from build123d import *

# Parameters (mm, degrees)
F0_R     = 3.175
F1_DEPTH = 35.56
F2_R     = 4.7625
F3_DEPTH = 3.81
F4_R     = 1.25


with BuildPart() as f1:
    # F0 (on Top) → F1 (new body)
    with BuildSketch(Plane.XY):
        Circle(F0_R)
    extrude(amount=-F1_DEPTH)

    # F2 (on Top) → F3 (join)
    with BuildSketch(Plane.XY):
        Circle(F2_R)
    extrude(amount=-F3_DEPTH)

    # F4
    f4_edges = [f1.edges().sort_by_distance(p)[0] for p in [
        (-3.175, 0, -35.56),
    ]]
    fillet(f4_edges, radius=F4_R)


solid = f1.part
Design review of the part built by this model. Coordinates are the model's own, in mm. A direction names the side the tool comes from. Round coordinates to 2 decimals unless told otherwise and drop trailing zeros. Order: outer loops, then holes, each group sorted by start corner. A loop starts at its lowest first (then second) coordinate and runs counter-clockwise, first axis right, second up. Notation, with made-up numbers: M 64,-19 L 110,-19 A3 ccw 110,-14 Z; hole C -23,51.5 d1. An arc over 180 degrees is marked long. Answer as CSV lines item,"result". Start each with the question number.
1) Add section C-C (z = -30). Give the boundary of the cut face in (x, y) (3 decimals), then the cut area to 3 significant figures.
2) Wall thickness on line 1 along Z through (x, y) = (0.25, 4); line 2 along X through (y, z) = (-2, -12.5); line 3 along X through (y, z) = (-1, -33): over which ranges is each line inside the solid? List them lowest first. Write a range as [from, to].
3) Tool access review of faces 1 (the face through (0, 0, 0)), 2 (the face through (-0.69, -3.1, -18.85)): name each direction out of +Z, -Z, +X, -X, +Y, -Y from which nothing blocks a thin tool from reaching the whole face with its end or side.
4) Add section D-D (z = -2.5). Give the boundary of the cut face in (x, y) (1 decimal).
5) For pin 1 Ø1.5 at (y, z) = (-1.5, -5.5) entering from -X; pin 2 Ø1.5 at (x, z) = (2, -22) entering from +Y; pin 3 Ø2 at (y, z) = (2.5, -5.5) entering from +X, all flat-tipped, find the tip position at first contact; note any pin that passes through.
Resolved:
1,outline,"C 0,0 d6.35"
1,area,"31.7 mm^2"
2,line 1,"[-3.81, 0]"
2,line 2,"[-2.47, 2.47]"
2,line 3,"[-3.01, 3.01]"
3,face 1,"+Z, +X, -X, +Y, -Y"
3,face 2,"-Z"
4,outline,"C 0,0 d9.5"
5,pin 1,"x = -3.09"
5,pin 2,"y = 2.92"
5,pin 3,"x = 2.8"
